Can you work these out from the model? Positions are in its coordinate system, mm. A direction names the side the tool comes from. Round coordinates to 2 decimals unless told otherwise and drop trailing zeros. Order: outer loops, then holes, each group sorted by start corner. A loop starts at its lowest first (then second) coordinate and runs counter-clockwise, first axis right, second up. Notation, with made-up numbers: (86.5, 64.5) -> (112.5, 64.5) arc R27 cw to (112.5, 98.5) -> close; hole circle Ø7 at (46, 9). An arc over 180 degrees is marked (long way). One line per item, written item: value.
```python
from build123d import *

# Parameters (mm, degrees)
F0_R      = 4
F1_DEPTH  = 25
F2_DEPTH  = 10
F3_SIZE   = 15
F4_R      = 10
F5_DEPTH  = 31
F6_W      = 20
F6_H      = 4
F7_DEPTH  = 24
F8_R      = 6
F9_DEPTH  = 31
F10_R     = 3
F11_DEPTH = 27


with BuildPart() as f1:
    # F0 (on Front) → F1 (new body, symmetric)
    with BuildSketch(Plane.XZ):
        with BuildLine():
            Line((-50, 0), (35, 0))
            Line((35, 0), (35, 27))
            Line((35, 27), (11, 27))
            Line((11, 27), (11, 24))
            Line((11, 24), (-1, 24))
            Line((-1, 24), (-1, 27))
            Line((-1, 27), (-14, 27))
            ThreePointArc((-14, 27), (-19.85235, 28.031038), (-25, 31))
            Line((-25, 31), (-50, 31))
            Line((-50, 31), (-50, 0))
        make_face()
        with Locations((-14, 12)):
            Circle(F0_R, mode=Mode.SUBTRACT)
        with Locations((23, 12)):
            Circle(F0_R, mode=Mode.SUBTRACT)
    extrude(amount=F1_DEPTH, both=True)

    # F0 (on Front) → F2 (join, symmetric)
    with BuildSketch(Plane.XZ):
        with BuildLine():
            Line((-1, 31), (-25, 31))
            ThreePointArc((-25, 31), (-19.85235, 28.031038), (-14, 27))
            Line((-14, 27), (-1, 27))
            Line((-1, 27), (-1, 31))
        make_face()
    extrude(amount=F2_DEPTH, both=True)

    # F3
    f3_edges = [f1.edges().sort_by_distance(p)[0] for p in [
        (-50, -25, 15.5),
        (-50, 25, 15.5),
    ]]
    chamfer(f3_edges, length=F3_SIZE)

    # F4 (on face) → F5 (cut)
    with BuildSketch(Plane.XY.offset(31)):
        with Locations((-50, 0)):
            Circle(F4_R)
    extrude(amount=-F5_DEPTH, mode=Mode.SUBTRACT)

    # F6 (on face) → F7 (join)
    with BuildSketch(Plane.YZ.offset(35)):
        with Locations((0, 29)):
            Rectangle(F6_W, F6_H)
    extrude(amount=-F7_DEPTH)

    # F8 (on face) → F9 (cut)
    with BuildSketch(Plane.XY.offset(31)):
        with Locations((-14.062501, 0)):
            Circle(F8_R)
        with Locations((23.372846, 0)):
            Circle(F8_R)
    extrude(amount=-F9_DEPTH, mode=Mode.SUBTRACT)

    # F10 (on face) → F11 (cut)
    with BuildSketch(Plane.XY.offset(24)):
        with Locations((5, 17.5)):
            Circle(F10_R)
        with Locations((5, -17.5)):
            Circle(F10_R)
    extrude(amount=-F11_DEPTH, mode=Mode.SUBTRACT)


solid = f1.part
```
Q1. I want a section at C-C on y = 0. List the corners of the cut face in (x, z) for me, plus the area to 3 significant figures.
Answers below:
outline: (-40, 0) -> (-20.06, 0) -> (-20.06, 31) -> (-40, 31) -> close; (-8.06, 0) -> (17.37, 0) -> (17.37, 31) -> (11, 31) -> (11, 24) -> (-1, 24) -> (-1, 31) -> (-8.06, 31) -> close; (29.37, 0) -> (35, 0) -> (35, 31) -> (29.37, 31) -> close
area: 1,500 mm^2
Q2. I want a section at A-A on y = -17.5. List the corners of the cut face in (x, z) for me (3 decimals), plus the area to 3 significant figures.
Answers below:
outline: (-42.5, 0) -> (2, 0) -> (2, 24) -> (-1, 24) -> (-1, 27) -> (-14, 27) arc R17.125 cw to (-25, 31) -> (-42.5, 31) -> close; (8, 0) -> (35, 0) -> (35, 27) -> (11, 27) -> (11, 24) -> (8, 24) -> close; hole circle Ø8 at (-14, 12); hole circle Ø8 at (23, 12)
area: 1,900 mm^2
Q3. Will these pins go through, and if not, where does the flat tip stop? pin 1 Ø10.5 at (x, y) = (-9, -14.5) entering from +Z; pin 2 Ø4.5 at (x, y) = (19, -21) entering from +Z; pin 3 Ø4 at (x, y) = (-20.5, -18) entering from +Z; pin 4 Ø1.5 at (y, z) = (-4, 14.5) entering from -X.
Answers below:
pin 1: z = 31
pin 2: z = 27
pin 3: z = 29.26
pin 4: x = -41.2
Q4. I want a section at B-B on x = 5. List the corners of the cut face in (y, z) for me, plus the area to 3 significant figures.
Answers below:
outline: (-25, 0) -> (-20.5, 0) -> (-20.5, 24) -> (-25, 24) -> close; (-14.5, 0) -> (14.5, 0) -> (14.5, 24) -> (-14.5, 24) -> close; (20.5, 0) -> (25, 0) -> (25, 24) -> (20.5, 24) -> close
area: 912 mm^2
Q5. We'd pull the mould along X, two halves only. Please class faces 5 (the face through (-7, -18, 27)), 6 (the face through (-43, 17, 16)), 7 (the face through (-8.52, -2.3, 15.72)): released by +X, released by -X, zero draft, split by the parting line, or undercut.
Answers below:
face 5: zero draft
face 6: released by -X
face 7: undercut
Q6. On a 3-axis mill with a long thin cutter (end or side, diameter ignored), from which of +Z, -Z, +X, -X, +Y, -Y can I reach the whole of each face in a straight line? I mean faces 1 (the face through (-7, 17, 27)), 2 (the face through (23, -10, 29)), 3 (the face through (23, -7, 31)), 4 (the face through (5, 0, 24)). Say none if no direction works.
Answers below:
face 1: +Z, +X, +Y
face 2: +Z, +X, -Y
face 3: +Z, +X, -X, +Y, -Y
face 4: +Z, +Y, -Y
Q7. Please list where these lines run through material, in increasing order: line 1 along X through (y, z) = (1, 7.5); line 2 along X through (y, z) = (2, 15.5); line 3 along Z through (x, y) = (23, -18).
Answers below:
line 1: -40.05 to -19.98, -8.15 to 17.46, 29.29 to 35
line 2: -40.2 to -19.72, -8.41 to 17.72, 29.03 to 35
line 3: 0 to 8, 16 to 27
Q8. I want a section at D-D on z = 15. List the corners of the cut face in (x, y) for me, plus the area to 3 significant figures.
Answers below:
outline: (-50, -10) -> (-35, -25) -> (-16.65, -25) -> (-16.65, -5.42) arc R6 cw to (-16.65, 5.42) -> (-16.65, 25) -> (-35, 25) -> (-50, 10) arc R10 cw to start; (-11.35, -25) -> (20.35, -25) -> (20.35, -5.19) arc R6 cw to (20.35, 5.19) -> (20.35, 25) -> (-11.35, 25) -> (-11.35, 5.35) arc R6 cw to (-11.35, -5.35) -> close; (25.65, -25) -> (35, -25) -> (35, 25) -> (25.65, 25) -> (25.65, 5.55) arc R6 cw to (25.65, -5.55) -> close; hole circle Ø6 at (5, -17.5); hole circle Ø6 at (5, 17.5)
area: 3,180 mm^2
